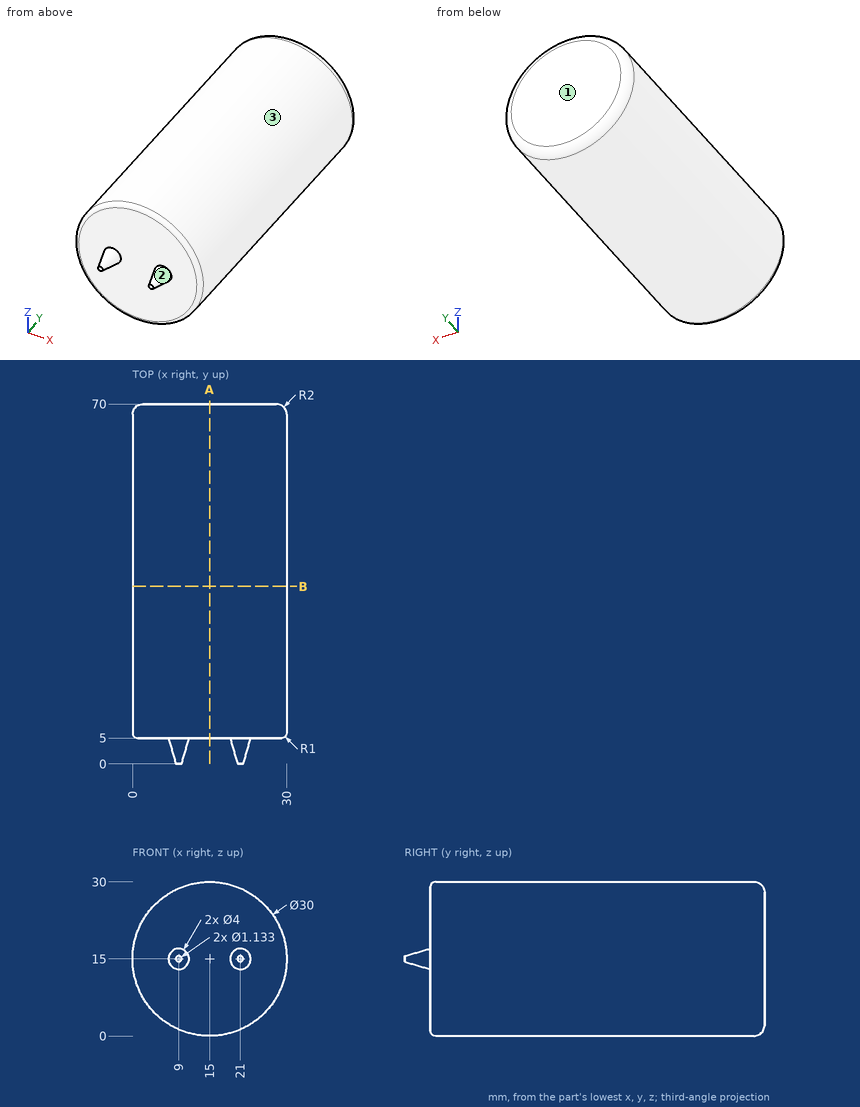
Input: dimensioned drawing with shaded views. Units: mm. Origin: part minimum x, y, z. Coordinates: 2 decimals unless noted, no trailing zeros. Order: outer loops, then holes, each group sorted by start corner. A loop starts at its lowest first (then second) coordinate and runs counter-clockwise, first axis right, second up. Notation, with made-up numbers: M -23.75,-25.75 L -14.75,-25.75 A8 cw -14.75,-19.75 Z; hole C 14,-17.5 d6. An arc over 180 degrees is marked long. Write each question's results on one line, items separated by ' | '. Start each with the question number.
Item 1: Line query: probe 1 along Y at (x, z) = (10.25, 23.75); probe 2 along X at (y, z) = (6, 23.75) (1 decimal); probe 3 along X at (y, z) = (25, 28.25) (1 decimal). Output: solid intervals per line, ascending.
Item 2: Cut plane A-A (x = 15). Return loops of the section in (y, z), and give its area (3 significant figures).
Item 3: First-contact query: pin 1 Ø10 at (y, z) = (17.5, 7) entering from +X; pin 2 Ø8 at (y, z) = (38.5, 24.5) entering from +X (1 decimal); pin 3 Ø10 at (x, z) = (22.5, 4) entering from -Y. Flat tips, straight axial feed; report the tip coordinate or a pass-through.
Item 4: Cut plane B-B (y = 34.5). Return loops of the section in (x, z), and give its area (3 significant figures).
Item 5: Draft query along X for the marked faces 1, 2 and 3. Return one class per face: pulls with the +X half, pulls with the -X half, needs draft (parallel to the pull), parting line crosses it, or undercut.
Checked values:
1) probe 1: y = 5 to 70 | probe 2: x = 2.8 to 27.2 | probe 3: x = 8 to 22
2) outline: M 5,1 A1 ccw 6,0 L 68,0 A2 ccw 70,2 L 70,28 A2 ccw 68,30 L 6,30 A1 ccw 5,29 Z | area: 1,950 mm2
3) pin 1: stops at x = 29.7 | pin 2: stops at x = 29 | pin 3: stops at y = 5
4) outline: C 15,15 d30 | area: 707 mm2
5) face 1: needs draft | face 2: undercut | face 3: parting line crosses it
